Check sheet for the modelled part. Datum: model origin and axes. Units: mm. Face numbers are marked on the shaded views. A direction names the side the tool comes from. Round coordinates to 2 decimals unless told otherwise and drop trailing zeros. Order: outer loops, then holes, each group sorted by start corner. A loop starts at its lowest first (then second) coordinate and runs counter-clockwise, first axis right, second up. Notation, with made-up numbers: (41.5, 53.5) -> (63.5, 53.5) arc R23 ccw to (63.5, 85.5) -> close; hole circle Ø7 at (-27.5, 20). An arc over 180 degrees is marked (long way). Use CSV: the item, a comma, the result in double quotes.
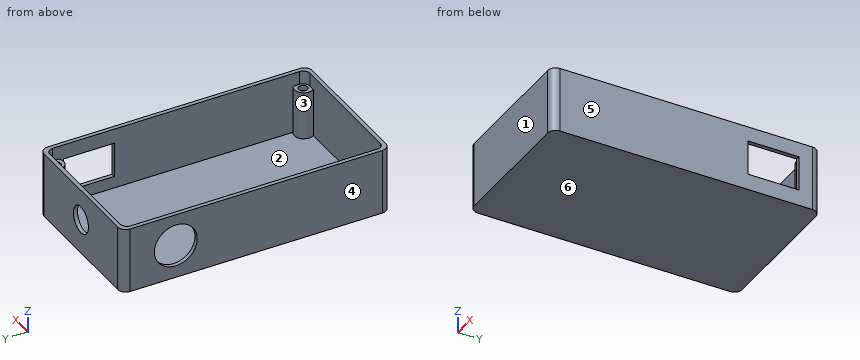
```python
from build123d import *

# Parameters (mm, degrees)
F0_W      = 55
F0_H      = 100
F1_DEPTH  = 24.5
F3_DEPTH  = 23
F4_R      = 5
F5_DEPTH  = 2
F6_R      = 8
F7_DEPTH  = 2
F8_R      = 3.5
F9_DEPTH  = 18
F10_R     = 1.65
F11_DEPTH = 2
F12_R     = 3
F13_R     = 2.5
F14_W     = 19
F14_H     = 13
F15_DEPTH = 2


with BuildPart() as f1:
    # F0 (on Top) → F1 (new body)
    with BuildSketch(Plane.XY):
        with Locations((27.5, 50)):
            Rectangle(F0_W, F0_H)
    extrude(amount=F1_DEPTH)

    # F2 (on face) → F3 (cut)
    with BuildSketch(Plane.XY.offset(24.5)):
        Polygon((27.5, 98.5), (1.5, 98.5), (1.5, 50), (1.5, 1.5), (27.5, 1.5), (53.5, 1.5), (53.5, 50), (53.5, 98.5), align=None)
    extrude(amount=-F3_DEPTH, mode=Mode.SUBTRACT)

    # F4 (on face) → F5 (cut)
    with BuildSketch(Plane(origin=(0, 100, 0), x_dir=(-1, 0, 0), z_dir=(0, 1, 0))):
        with Locations((-27.5, 13)):
            Circle(F4_R)
    extrude(amount=-F5_DEPTH, mode=Mode.SUBTRACT)

    # F6 (on face) → F7 (cut)
    with BuildSketch(Plane(origin=(0, 0, 0), x_dir=(0, -1, 0), z_dir=(-1, 0, 0))):
        with Locations((-80, 12.5)):
            Circle(F6_R)
    extrude(amount=-F7_DEPTH, mode=Mode.SUBTRACT)

    # F8 (on face) → F9 (join)
    with BuildSketch(Plane.XY.offset(1.5)):
        with Locations((3.5, 96.5)):
            Circle(F8_R)
        with Locations((51.5, 96.5)):
            Circle(F8_R)
        with Locations((51.5, 3.5)):
            Circle(F8_R)
        with Locations((3.5, 3.5)):
            Circle(F8_R)
    extrude(amount=F9_DEPTH)

    # F10 (on face) → F11 (cut)
    with BuildSketch(Plane.XY.offset(19.5)):
        with Locations((4, 96)):
            Circle(F10_R)
        with Locations((4, 4)):
            Circle(F10_R)
        with Locations((51, 96)):
            Circle(F10_R)
        with Locations((51, 4)):
            Circle(F10_R)
    extrude(amount=-F11_DEPTH, mode=Mode.SUBTRACT)

    # F12
    f12_edges = [f1.edges().sort_by_distance(p)[0] for p in [
        (0, 100, 12.25),
        (55, 100, 12.25),
        (0, 0, 12.25),
        (55, 0, 12.25),
    ]]
    fillet(f12_edges, radius=F12_R)

    # F13
    f13_edges = [f1.edges().sort_by_distance(p)[0] for p in [
        (1.5, 98.5, 22),
        (53.5, 98.5, 22),
        (1.5, 1.5, 22),
        (53.5, 1.5, 22),
    ]]
    fillet(f13_edges, radius=F13_R)

    # F14 (on face) → F15 (cut)
    with BuildSketch(Plane.YZ.offset(55)):
        with Locations((82.5, 12.5)):
            Rectangle(F14_W, F14_H)
    extrude(amount=-F15_DEPTH, mode=Mode.SUBTRACT)


solid = f1.part
```
Q1. Mould release check, pull along X, two halves, no side actions. Record for the marked faces 3, 4, 5 and 6: pulls with the +X half, pulls with the -X half, needs draft (parallel to the pull), parting line crosses it, or undercut.
Result sheet:
face 3,"undercut"
face 4,"pulls with the -X half"
face 5,"pulls with the +X half"
face 6,"needs draft"
Q2. Scan lines: L1, parallel to Y at x = 30.5, z = 22.5; L2, parallel to X at y = 72, z = 9.75; L3, parallel to Z at x = 27.5, y = 99.1. Record each from-to range of solid material in increasing order.
Result sheet:
L1,"y = 0 to 1.5, 98.5 to 100"
L2,"x = 0 to 1.5, 53.5 to 55"
L3,"z = 0 to 8, 18 to 24.5"
Q3. Go/stop test with flat-tipped pins: pin 1 (4.5 mm diameter, centred on x = 4, y = 96, fed in from +Z); pin 2 (1.2 mm diameter, centred on x = 54, z = 10, fed in from -Y); pin 3 (2 mm diameter, centred on x = 51, y = 96, fed in from +Z). Record where each tip stops, or that it passes through.
Result sheet:
pin 1,"stops at z = 19.5"
pin 2,"stops at y = 0.35"
pin 3,"stops at z = 17.5"
Q4. Access from +Z, -Z, +X, -X, +Y, -Y to the whole of each face (thin tool, end or side, straight path). Record for the marked faces 1 and 2.
Result sheet:
face 1,"+Z, -Z, +X, -X, -Y"
face 2,"+Z"
Q5. Sectioned sample at A-A, the plane x = 27.5. Enter the section's corners in (y, z), then the cut area to 3 significant figures.
Result sheet:
outline,"(0, 0) -> (100, 0) -> (100, 8) -> (98.5, 8) -> (98.5, 1.5) -> (1.5, 1.5) -> (1.5, 24.5) -> (0, 24.5) -> close; (98.5, 18) -> (100, 18) -> (100, 24.5) -> (98.5, 24.5) -> close"
area,"204 mm^2"
Q6. Sectioned sample at B-B, the plane y = 80. Enter the section's corners in (x, z), then the cut area to 3 significant figures.
Result sheet:
outline,"(0, 0) -> (55, 0) -> (55, 6) -> (53.5, 6) -> (53.5, 1.5) -> (1.5, 1.5) -> (1.5, 4.5) -> (0, 4.5) -> close; (0, 20.5) -> (1.5, 20.5) -> (1.5, 24.5) -> (0, 24.5) -> close; (53.5, 19) -> (55, 19) -> (55, 24.5) -> (53.5, 24.5) -> close"
area,"108 mm^2"
Q7. Sectioned sample at D-D, the plane y = 28. Enter the section's corners in (x, z), then the cut area to 4 significant figures.
Result sheet:
outline,"(0, 0) -> (55, 0) -> (55, 24.5) -> (53.5, 24.5) -> (53.5, 1.5) -> (1.5, 1.5) -> (1.5, 24.5) -> (0, 24.5) -> close"
area,"151.5 mm^2"
Q8. Sectioned sample at C-C, the plane z = 10.25. Enter the section's corners in (x, y), then the cut area to 3 significant figures.
Result sheet:
outline,"(0, 3) arc R3 ccw to (3, 0) -> (52, 0) arc R3 ccw to (55, 3) -> (55, 73) -> (53.5, 73) -> (53.5, 6.37) arc R3.5 ccw to (48.63, 1.5) -> (6.37, 1.5) arc R3.5 ccw to (1.5, 6.37) -> (1.5, 72.32) -> (0, 72.32) -> close; (0, 87.68) -> (1.5, 87.68) -> (1.5, 93.63) arc R3.5 ccw to (6.37, 98.5) -> (23.32, 98.5) -> (23.32, 100) -> (3, 100) arc R3 ccw to (0, 97) -> close; (31.68, 98.5) -> (48.63, 98.5) arc R3.5 ccw to (53.5, 93.63) -> (53.5, 92) -> (55, 92) -> (55, 97) arc R3 ccw to (52, 100) -> (31.68, 100) -> close"
area,"491 mm^2"
